```python
from build123d import *

# Parameters (mm, degrees)
F0_W     = 96.026704
F0_H     = 88.803456
F1_DEPTH = 25.4
F2_R     = 16.580818
F3_DEPTH = 25.4
F5_DEPTH = 88.804455


with BuildPart() as f1:
    # F0 (on Front) → F1 (new body)
    with BuildSketch(Plane.XZ):
        Rectangle(F0_W, F0_H)
    extrude(amount=F1_DEPTH)

    # F2 (on face) → F3 (join)
    with BuildSketch(Plane.XZ.offset(25.4)):
        with Locations((1.380454, 2.939289)):
            Circle(F2_R)
    extrude(amount=F3_DEPTH)

    # F4 (on face) → F5 (cut, through all)
    with BuildSketch(Plane(origin=(0, 0, -44.401728), x_dir=(1, 0, 0), z_dir=(0, 0, -1))):
        Polygon((17.961273, 50.8), (-15.200364, 50.8), (17.961273, 25.4), align=None)
    extrude(amount=-F5_DEPTH, mode=Mode.SUBTRACT)


solid = f1.part
```
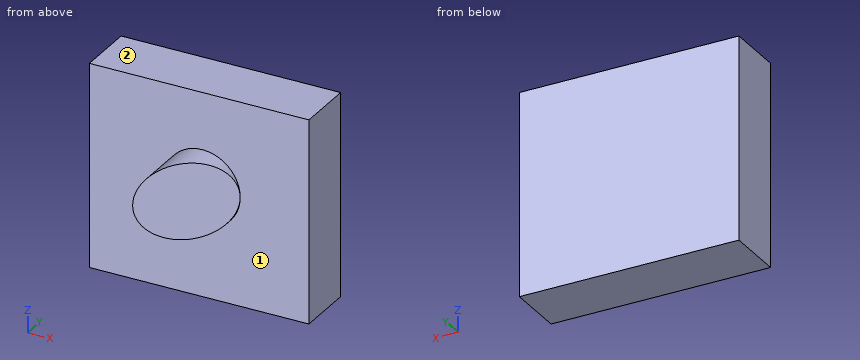
Work out the finished part from the listing and answer in its coordinate system (mm). Face numbers are marked on the shaded views. A direction names the side the tool comes from. Give positions to 0.01 mm unless a question says otherwise; leave off trailing zeros. Write each loop counter-clockwise with the first axis right and the second up, starting at its lowest first coordinate (ties: lowest second). Pieces come first, ordered by that corner, then holes.
(1) A flat-ended cylindrical pin translates along its axis: pin 1 Ø10 at (x, z) = (-24, -24) entering from -Y. Find the tip coordinate at first contact, or state that the pin passes through.
Final values:
pin 1: stops at y = -25.4
(2) Which of the six approach directions +Z, -Z, +X, -X, +Y, -Y give full straight-line access (tool end or side, diameter ignored) to the marked faces 1 and 2?
Final values:
face 1: -Y
face 2: +Z, +X, -X, +Y, -Y
(3) Straight lines are drawn through the part: line 1 (Y direction, x = -17, z = -19.5); line 2 (X direction, y = -42, z = 12.5); line 3 (X direction, y = -31, z = -9.5). For each, find the intervals that lie inside material, in ascending order.
Final values:
line 1: y = -25.4 to 0
line 2: x = -12.17 to -3.71
line 3: x = -9.58 to 10.65
(4) The part is cut by section A-A on x = 31. Write down the section's boundary in (y, z), plus the area to 3 significant figures.
Final values:
outline: (-25.4, -44.4) - (0, -44.4) - (0, 44.4) - (-25.4, 44.4) - close
area: 2,260 mm2
(5) The part is cut by section D-D on z = -20. Write down the section's boundary in (x, y), plus the area to 3 significant figures.
Final values:
outline: (-48.01, -25.4) - (48.01, -25.4) - (48.01, 0) - (-48.01, 0) - close
area: 2,440 mm2
(6) The part is cut by section C-C on y = -43.5. Write down the section's boundary in (x, z), plus the area to 3 significant figures.
Final values:
outline: (-5.67, -12.07) - (-5.67, 17.95) arc R16.58 ccw to start
area: 205 mm2
(7) The part is cut by section B-B on z = -6.5. Write down the section's boundary in (x, y).
Final values:
outline: (-48.01, -25.4) - (-12.25, -25.4) - (-12.25, -48.54) - (15.01, -27.66) - (15.01, -25.4) - (48.01, -25.4) - (48.01, 0) - (-48.01, 0) - close
